Here's how the part is built. I have some questions about the finished solid (model axes, mm). A direction names the side the tool comes from. Give positions to 0.01 mm unless a question says otherwise; leave off trailing zeros. Loops run counter-clockwise (first coordinate to the right, second up) from the corner with the lowest first, then second, coordinate; pieces in that order, holes last.
Q1. Suppose I cut it at A-A (z = 0). List the corners of the cut face in (x, y) for me, and give its area (3 significant figures).
Q2. Suppose I cut it at C-C (x = 45.5). List the corners of the cut face in (y, z) for me, and give its area (3 significant figures).
Q3. Thinking about a two-plate mould opening in Z: for faces 1 (the face through (1, 0, -1)), 2 (the face through (19.52, 9.86, 62)), 3 (the face through (-34.063, 2.535, -23.114)), which applies, pulls with the +Z half, pulls with the -Z half, needs draft (parallel to the pull), parting line crosses it, or undercut?
Q4. Suppose I cut it at B-B (z = 43). List the corners of the cut face in (x, y) for me.
Q5. I'm going to push flat-ended pins straight in: P1, Ø4, axis at y = 5, z = -11.5, coming from the +X side; P2, Ø8, axis at y = 15, z = -38.5, coming from the -X side; P3, Ø4, axis at y = 17.5, z = -10, coming from the +X side; P4, Ø11.5, axis at x = -37.33, z = -29.39, coming from the +Y side. Where does each tip first touch, or does it pass through?
Q6. Suppose I cut it at D-D (y = 7.5). List the corners of the cut face in (x, z) for me, and give its area (3 significant figures).
Q7. I need wall thicknesses on probe 1 along X at (y, z) = (11.5, 0); probe 2 along Y at (x, z) = (-21, 15); probe 3 along Z at (x, y) = (2.5, 16.25). Which ranges of each line are inside material? Lowest first, please.
Q8. For faces 4 (the face through (14.7, 20, -53.3)), 5 (the face through (1, 5, -1)), which set-ups out of +Z, -Z, +X, -X, +Y, -Y let a thin tool reach every point of the face, with its end or its side?
```python
from build123d import *

# Parameters (mm, degrees)
SKETCH1_R                 = 65
BOSS_EXTRUDE1_DEPTH       = 20
SKETCH2_R                 = 55
CUT_EXTRUDE1_DEPTH        = 15
F_1_0MM_DOWEL_HOLE1_D     = 14.15
F_1_0MM_DOWEL_HOLE1_DEPTH = 8.14891112
F_1_0MM_DOWEL_HOLE1_TIP   = 4.25108888


with BuildPart() as part:
    # Sketch1 → Boss-Extrude1 (new body)
    with BuildSketch(Plane(origin=(0, 0, 0), x_dir=(1, 0, 0), z_dir=(0, 1, 0))):
        with Locations(Location((0, 0, 0), (0, 0, 270))):
            Circle(SKETCH1_R)
    extrude(amount=BOSS_EXTRUDE1_DEPTH)

    # Sketch2 → Cut-Extrude1 (cut)
    with BuildSketch(Plane(origin=(0, 20, 0), x_dir=(1, 0, 0), z_dir=(0, 1, 0))):
        with Locations(Location((0, 0, 0), (0, 0, 270))):
            Circle(SKETCH2_R)
    extrude(amount=-CUT_EXTRUDE1_DEPTH, mode=Mode.SUBTRACT)

    # Ø1.0mm Dowel Hole1
    with Locations(Plane(origin=(0, 0, 0), x_dir=(-1, 0, 0), z_dir=(0, -1, 0))):
        with Locations((37.328017274, 29.390801732), (6.7891723, -47.022412098), (-44.117189574, 17.631610366)):
            Hole(F_1_0MM_DOWEL_HOLE1_D / 2, depth=F_1_0MM_DOWEL_HOLE1_DEPTH)
            with Locations((0, 0, -(F_1_0MM_DOWEL_HOLE1_DEPTH + F_1_0MM_DOWEL_HOLE1_TIP / 2))):  # 118° drill point
                Cone(0, F_1_0MM_DOWEL_HOLE1_D / 2, F_1_0MM_DOWEL_HOLE1_TIP, mode=Mode.SUBTRACT)


solid = part.part
```
Solutions:
1. outline: (-65, 0) - (65, 0) - (65, 20) - (55, 20) - (55, 5) - (-55, 5) - (-55, 20) - (-65, 20) - close
1. area: 950 mm2
2. outline: (0, -46.42) - (20, -46.42) - (20, -30.9) - (5, -30.9) - (5, -24.57) - (0, -24.57) - close; (0, -10.69) - (5, -10.69) - (5, 30.9) - (20, 30.9) - (20, 46.42) - (0, 46.42) - close
2. area: 860 mm2
3. face 1: needs draft
3. face 2: parting line crosses it
3. face 3: undercut
4. outline: (-48.74, 0) - (-12.61, 0) - (-12.61, 5) - (-34.29, 5) - (-34.29, 20) - (-48.74, 20) - close; (-0.97, 0) - (48.74, 0) - (48.74, 20) - (34.29, 20) - (34.29, 5) - (-0.97, 5) - close
5. P1: stops at x = 64.3
5. P2: stops at x = -55.09
5. P3: stops at x = 64.51
5. P4: passes through
6. outline: circle Ø130 at (0, 0); hole circle Ø110 at (0, 0)
6. area: 3,770 mm2
7. probe 1: x = -65 to -55, 55 to 65
7. probe 2: y = 0 to 5
7. probe 3: z = -64.95 to -54.94, 54.94 to 64.95
8. face 4: +Z, -Z, +X, -X, +Y
8. face 5: +Y
